```python
from build123d import *

# Parameters (mm, degrees)
BOSS_EXTRUDE1_DEPTH     = 50
CUT_EXTRUDE1_DEPTH      = 60.332090981
SKETCH3_W               = 15
SKETCH3_H               = 3.3
CUT_EXTRUDE2_DEPTH      = 60.332090981
CUT_EXTRUDE4_DEPTH      = 60.332090981
CUT_EXTRUDE4_DEPTH_BACK = 10
FILLET1_R               = 2
FILLET2_R               = 5
CUT_EXTRUDE5_DEPTH      = 60.332090981
CUT_EXTRUDE5_DEPTH_BACK = 60.332090981
SKETCH7_R               = 2
FILLET3_R               = 4


with BuildPart() as part:
    # Sketch1 → Boss-Extrude1 (new body)
    with BuildSketch(Plane.XY):
        Polygon((2.5, 7.92), (4.58, 10), (5.287106781, 10.707106781), (10.707106781, 10.707106781), (10.707106781, 5.287106781), (10, 4.58), (7.92, 2.5), (5.92, 2.5), (5.92, -2.5), (7.92, -2.5), (10, -4.58), (10.707106781, -5.287106781), (10.707106781, -7.287106781), (13.707106781, -7.287106781), (13.707106781, 10.707106781), (28.707106781, 10.707106781), (28.707106781, 14.007106781), (13.707106781, 14.007106781), (-7.287106781, 14.007106781), (-7.287106781, 10.707106781), (-5.287106781, 10.707106781), (-4.58, 10), (-2.5, 7.92), (-2.5, 5.92), (2.5, 5.92), align=None)
    boss_extrude1 = extrude(amount=BOSS_EXTRUDE1_DEPTH)

    # Sketch2 → Cut-Extrude1 (cut, through all)
    with BuildSketch(Plane.XY):
        Polygon((0, 0), (18.478629357, 0), (18.478629357, -9.938314006), (0, -9.42769987), align=None)
    extrude(amount=CUT_EXTRUDE1_DEPTH, mode=Mode.SUBTRACT)

    # Mirror1: Boss-Extrude1 across plane
    add(boss_extrude1.mirror(Plane.ZX))

    # Sketch3 → Cut-Extrude2 (cut, through all)
    with BuildSketch(Plane.XY):
        with Locations((21.207106781, -12.357106781)):
            Rectangle(SKETCH3_W, SKETCH3_H)
    extrude(amount=CUT_EXTRUDE2_DEPTH, mode=Mode.SUBTRACT)

    # Sketch6 → Cut-Extrude4 (cut, two sides: drawn at the far end of the back side and taken through both)
    with BuildSketch(Plane.XY.offset(-CUT_EXTRUDE4_DEPTH_BACK)):
        Polygon((-5.287106781, 10.707106781), (-4.287106781, 10.707106781), (-2.5, 8.92), (-2.5, 7.92), align=None)
        Polygon((2.5, 7.92), (2.5, 8.92), (4.287106781, 10.707106781), (5.287106781, 10.707106781), align=None)
        Polygon((7.92, 2.5), (8.92, 2.5), (10.707106781, 4.287106781), (10.707106781, 5.287106781), align=None)
        Polygon((7.92, -2.5), (10.707106781, -5.287106781), (10.707106781, -4.287106781), (8.92, -2.5), align=None)
        Polygon((2.5, -7.92), (5.287106781, -10.707106781), (4.287106781, -10.707106781), (2.5, -8.92), align=None)
        Polygon((-5.287106781, -10.707106781), (-2.5, -7.92), (-2.5, -8.92), (-4.287106781, -10.707106781), align=None)
    extrude(amount=CUT_EXTRUDE4_DEPTH + CUT_EXTRUDE4_DEPTH_BACK, mode=Mode.SUBTRACT)

    # Fillet1
    # the kernel refuses this fillet: 2 mm, written as the material it adds along each edge
    with BuildSketch(Plane(origin=(10.707106781, 10.707106781, 0), x_dir=(0, -1, 0), z_dir=(0, 0, 1)), Plane(origin=(10.707106781, -10.707106781, 0), x_dir=(-1, 0, 0), z_dir=(0, 0, 1))) as fillet1_piece_1:
        with BuildLine():
            CenterArc((FILLET1_R, -FILLET1_R), FILLET1_R, 90, 90)
            Line((0, -FILLET1_R), (0, 0))
            Line((0, 0), (FILLET1_R, 0))
        make_face()
    extrude(amount=50)
    # the kernel refuses this fillet: 2 mm, written as the material it takes off along each edge
    with BuildSketch(Plane(origin=(13.707106781, -14.007106781, -5), x_dir=(-1, 0, 0), z_dir=(0, 0, 1)), Plane(origin=(5.92, 2.5, -5), x_dir=(1, 0, 0), z_dir=(0, 0, 1)), Plane(origin=(2.5, 5.92, -5), x_dir=(-1, 0, 0), z_dir=(0, 0, 1)), Plane(origin=(-2.5, 5.92, -5), x_dir=(0, 1, 0), z_dir=(0, 0, 1)), Plane(origin=(-7.287106781, 10.707106781, -5), x_dir=(0, 1, 0), z_dir=(0, 0, 1)), Plane(origin=(28.707106781, 10.707106781, -5), x_dir=(-1, 0, 0), z_dir=(0, 0, 1)), Plane(origin=(5.92, -2.5, -5), x_dir=(0, 1, 0), z_dir=(0, 0, 1)), Plane(origin=(2.5, -5.92, -5), x_dir=(0, -1, 0), z_dir=(0, 0, 1)), Plane(origin=(-2.5, -5.92, -5), x_dir=(1, 0, 0), z_dir=(0, 0, 1)), Plane(origin=(-7.287106781, -10.707106781, -5), x_dir=(1, 0, 0), z_dir=(0, 0, 1)), Plane(origin=(-7.287106781, -14.007106781, -5), x_dir=(0, 1, 0), z_dir=(0, 0, 1))) as fillet1_2_piece_1:
        with BuildLine():
            CenterArc((FILLET1_R, -FILLET1_R), FILLET1_R, 90, 90)
            Line((0, -FILLET1_R), (0, 0))
            Line((0, 0), (FILLET1_R, 0))
        make_face()
    extrude(amount=60, mode=Mode.SUBTRACT)

    # Fillet2
    fillet2_edges = [part.edges().sort_by_distance(p)[0] for p in [
        (13.707106781, 10.707106781, 25),
    ]]
    fillet(fillet2_edges, radius=FILLET2_R)

    # Sketch7 → Cut-Extrude5 (cut, two sides: drawn at the far end of the back side and taken through both)
    with BuildSketch(Plane(origin=(0, 0, 0), x_dir=(1, 0, 0), z_dir=(0, 1, 0)).offset(-CUT_EXTRUDE5_DEPTH_BACK)):
        with Locations(Location((21.207106781, -40, 0), (0, 0, 270))):
            Circle(SKETCH7_R)
        with Locations(Location((21.207106781, -25, 0), (0, 0, 270))):
            Circle(SKETCH7_R)
        with Locations(Location((21.207106781, -10, 0), (0, 0, 270))):
            Circle(SKETCH7_R)
    extrude(amount=CUT_EXTRUDE5_DEPTH + CUT_EXTRUDE5_DEPTH_BACK, mode=Mode.SUBTRACT)

    # Fillet3
    # the kernel refuses this fillet: 4 mm, written as the material it takes off along each edge
    with BuildSketch(Plane(origin=(-10.5, -5.92, 0), x_dir=(0, -1, 0), z_dir=(1, 0, 0))) as fillet3_piece_1_section:
        with BuildLine():
            CenterArc((FILLET3_R, -FILLET3_R), FILLET3_R, 90, 90)
            Line((0, -FILLET3_R), (0, 0))
            Line((0, 0), (FILLET3_R, 0))
        make_face()
    fillet3_piece_1 = extrude(amount=21, mode=Mode.PRIVATE)
    fillet3_piece_1 = split(fillet3_piece_1, bisect_by=Plane(origin=(2.5, -6.766631822, 0.880672942), z_dir=(-1, 0, 0)), keep=Keep.TOP, mode=Mode.PRIVATE)
    add(fillet3_piece_1, mode=Mode.SUBTRACT)
    with BuildSketch(Plane(origin=(-10.5, -5.92, 0), x_dir=(0, -1, 0), z_dir=(1, 0, 0))) as fillet3_piece_2_section:
        with BuildLine():
            CenterArc((FILLET3_R, -FILLET3_R), FILLET3_R, 90, 90)
            Line((0, -FILLET3_R), (0, 0))
            Line((0, 0), (FILLET3_R, 0))
        make_face()
    fillet3_piece_2 = extrude(amount=21, mode=Mode.PRIVATE)
    fillet3_piece_2 = split(fillet3_piece_2, bisect_by=Plane(origin=(2.799453379, -9.219453379, 0.025268376), z_dir=(-0.7071067811865467, -0.7071067811865485, 0)), keep=Keep.TOP, mode=Mode.PRIVATE)
    add(fillet3_piece_2, mode=Mode.SUBTRACT)
    with BuildSketch(Plane(origin=(5.92, -10.5, 0), x_dir=(1, 0, 0), z_dir=(0, 1, 0))) as fillet3_piece_3_section:
        with BuildLine():
            CenterArc((FILLET3_R, -FILLET3_R), FILLET3_R, 90, 90)
            Line((0, -FILLET3_R), (0, 0))
            Line((0, 0), (FILLET3_R, 0))
        make_face()
    fillet3_piece_3 = extrude(amount=21, mode=Mode.PRIVATE)
    fillet3_piece_3 = split(fillet3_piece_3, bisect_by=Plane(origin=(6.766631909, -2.5, 0.880672877), z_dir=(0, 1, 0)), keep=Keep.TOP, mode=Mode.PRIVATE)
    fillet3_piece_3 = split(fillet3_piece_3, bisect_by=Plane(origin=(6.766631909, 2.5, 0.880672877), z_dir=(0, -1, 0)), keep=Keep.TOP, mode=Mode.PRIVATE)
    add(fillet3_piece_3, mode=Mode.SUBTRACT)
    with BuildSketch(Plane(origin=(5.92, -10.5, 0), x_dir=(1, 0, 0), z_dir=(0, 1, 0))) as fillet3_piece_4_section:
        with BuildLine():
            CenterArc((FILLET3_R, -FILLET3_R), FILLET3_R, 90, 90)
            Line((0, -FILLET3_R), (0, 0))
            Line((0, 0), (FILLET3_R, 0))
        make_face()
    fillet3_piece_4 = extrude(amount=21, mode=Mode.PRIVATE)
    fillet3_piece_4 = split(fillet3_piece_4, bisect_by=Plane(origin=(9.219453379, -2.799453379, 0.025268376), z_dir=(0.7071067811865552, 0.7071067811865398, 0)), keep=Keep.TOP, mode=Mode.PRIVATE)
    fillet3_piece_4 = split(fillet3_piece_4, bisect_by=Plane(origin=(6.519817793, 0.099817793, 0.025268376), z_dir=(0.7071067811865552, -0.7071067811865398, 0)), keep=Keep.TOP, mode=Mode.PRIVATE)
    add(fillet3_piece_4, mode=Mode.SUBTRACT)
    with BuildSketch(Plane(origin=(-10.5, 5.92, 0), x_dir=(0, 1, 0), z_dir=(1, 0, 0))) as fillet3_piece_5_section:
        with BuildLine():
            CenterArc((FILLET3_R, FILLET3_R), FILLET3_R, 180, 90)
            Line((0, FILLET3_R), (0, 0))
            Line((0, 0), (FILLET3_R, 0))
        make_face()
    fillet3_piece_5 = extrude(amount=21, mode=Mode.PRIVATE)
    fillet3_piece_5 = split(fillet3_piece_5, bisect_by=Plane(origin=(2.5, 6.766633177, 0.880671903), z_dir=(-1, 0, 0)), keep=Keep.TOP, mode=Mode.PRIVATE)
    add(fillet3_piece_5, mode=Mode.SUBTRACT)
    with BuildSketch(Plane(origin=(-10.5, 5.92, 0), x_dir=(0, 1, 0), z_dir=(1, 0, 0))) as fillet3_piece_6_section:
        with BuildLine():
            CenterArc((FILLET3_R, FILLET3_R), FILLET3_R, 180, 90)
            Line((0, FILLET3_R), (0, 0))
            Line((0, 0), (FILLET3_R, 0))
        make_face()
    fillet3_piece_6 = extrude(amount=21, mode=Mode.PRIVATE)
    fillet3_piece_6 = split(fillet3_piece_6, bisect_by=Plane(origin=(2.799453379, 9.219453379, 0.025268376), z_dir=(-0.7071067811865467, 0.7071067811865485, 0)), keep=Keep.TOP, mode=Mode.PRIVATE)
    add(fillet3_piece_6, mode=Mode.SUBTRACT)


solid = part.part
```
Can you work these out from the model? Positions are in its coordinate system, mm. A direction names the side the tool comes from. Give positions to 0.01 mm unless a question says otherwise; leave off trailing zeros. Order: outer loops, then holes, each group sorted by start corner. A loop starts at its lowest first (then second) coordinate and runs counter-clockwise, first axis right, second up. Notation, with made-up numbers: M 70.5,-32 L 101.5,-32 A31 cw 101.5,-5 Z; hole C 18,18.5 d6. An arc over 180 degrees is marked long. Write item = value, one per line. Start each with the question number.
Q1. Suppose I cut it at A-A (x = 25.5). Write out the boundary of the cut face in (y, z).
Q2. I need wall thicknesses on probe 1 along X at (y, z) = (-7.75, 19); probe 2 along Y at (x, z) = (9, 38); probe 3 along Y at (x, z) = (5, 11). Which ranges of each line are inside material? Lowest first, please. Write a range as [from, to].
Q3. For faces 1 (the cylindrical face through (10.106, -10.137, 24.65)), 2 (the cylindrical face through (-6.72, 11.31, 24.65)), 3 (the flat face through (24, 10.707, 25)), 4 (the flat face through (28.707, 13, 25)), 5 (the cylindrical face through (19.43, 12.33, 10.92)), which set-ups out of +Z, -Z, +X, -X, +Y, -Y let a thin tool reach every point of the face, with its end or its side?
Q4. We'd pull the mould along Y, two halves only. Please class faces 6 (the cylindrical face through (19.99, 12.334, 23.413)), 7 (the cylindrical face through (28.11, 11.28, 24.65)), 8 (the flat face through (3.41, -9.83, 24.65)): pulls with the +Y half, pulls with the -Y half, needs draft (parallel to the pull), parting line crosses it, or undercut.
Q5. Will these pins go through, and if not, where does the flat tip stop? pin 1 Ø2 at (y, z) = (-7, 29) entering from -X; pin 2 Ø12 at (y, z) = (0, 38) entering from +X; pin 3 Ø4.5 at (x, z) = (21.21, 10) entering from -Y; pin 4 Ø12 at (x, y) = (3, 8) entering from -Z.
Check result:
q1.outline = M 10.71,0 L 14.01,0 L 14.01,50 L 10.71,50 Z
q2.probe_1 = [-2.49, 2.49], [10.71, 13.71]
q2.probe_2 = [-14.01, -10.69], [-2.58, 2.58], [10.69, 14.01]
q2.probe_3 = [-14.01, -10.71], [10.71, 14.01]
q3.face_1 = +Z, -Z
q3.face_2 = +Z, -Z, -X
q3.face_3 = +Z, -Z, +X, -Y
q3.face_4 = +Z, -Z, +X, +Y, -Y
q3.face_5 = +Y, -Y
q4.face_6 = needs draft
q4.face_7 = pulls with the -Y half
q4.face_8 = undercut
q5.pin_1 = -2.5
q5.pin_2 = 13.72
q5.pin_3 = 10.71
q5.pin_4 = 0
